Autodesk Inventor part; units mm, degrees
ref_plane "YZ Plane" through (0, 0, 0) normal (1, 0, 0) x (0, 1, 0)
ref_plane "XZ Plane" through (0, 0, 0) normal (0, 1, 0) x (-1, 0, 0)
ref_plane "XY Plane" through (0, 0, 0) normal (0, 0, 1) x (1, 0, 0)
sketch "Sketch1" plane through (0, 0, 0) normal (0, 0, 1) x (1, 0, 0)
  line L0 (-4.3614, 7.1036) -> (6.1386, 7.1036)
  line L1 (6.1386, 7.1036) -> (6.1386, -5.3964)
  line L2 (-4.3614, -5.3964) -> (-4.3614, 7.1036)
  line L3 (-4.3614, -5.3964) -> (-17.0614, -5.3964)
  line L4 (-4.3614, -5.3964) -> (8.3386, -5.3964) construction
  line L5 (-17.0614, -5.3964) -> (-17.0614, 12.1836)
  line L6 (-17.0614, 12.1836) -> (18.8386, 12.1836)
  line L7 (18.8386, 12.1836) -> (18.8386, -5.3964)
  line L8 (18.8386, -5.3964) -> (6.1386, -5.3964)
  point P0 (0, 0)
  dimension "d0" = 10.5
  dimension "d1" = 12.5
  dimension "d2" = 12.7
  dimension "d3" = 180
  dimension "d6" = 12.7
  dimension "d9" = 5.08
extrude "Extrusion1" add sketch "Sketch1" along normal blind 15
sketch "Sketch2" plane through (6.1386, -5.3964, 0) normal (0, -1, 0) x (1, 0, 0)
  circle A0 centre (6.35, 7.5) radius 3.175
  circle A1 centre (-16.85, 7.5) radius 3.175
  line L0 (0, 0) -> (12.7, 0)
  line L1 (-23.2, 0) -> (-23.2, 15)
  line L2 (-23.2, 15) -> (-10.5, 15)
  point P0 (-6.1386, 0)
  dimension "d12" = 6.35
  dimension "d13" = 6.35
  dimension "d14" = 7.5
  dimension "d15" = 6.35
  dimension "d16" = 6.35
  dimension "d17" = 7.5
extrude "Extrusion2" cut sketch "Sketch2" against normal blind 21.5125
properties part number "motor mount"
For this review, take the finished solid that the model builds, in its own axes (mm). A direction names the side the tool comes from. Round coordinates to 2 decimals unless told otherwise and drop trailing zeros. Write each loop counter-clockwise with the first axis right and the second up, starting at its lowest first coordinate (ties: lowest second). Pieces come first, ordered by that corner, then holes. Notation, with made-up numbers: (48, 29) - (52, 29) arc R9 ccw to (52, 41) - close; hole circle Ø6 at (10, 34). An arc over 180 degrees is marked (long way). Answer as a JSON object with one key per item and string values.
1. Draft analysis for pull direction Z (two halves, no side actions). For faces 3 (the face through (1, 12.184, 7)), 4 (the face through (0.6, 7.4, 15)), 5 (the face through (-7.78, 3.27, 6.28)), state which applies: +Z half, -Z half, draft (parallel to the pull), parting line (faces both ways), or undercut.
Response values:
{"face 3": "draft", "face 4": "+Z half", "face 5": "undercut"}
2. We need section A-A on y = 3.5. Give the boundary of the cut face in (x, z) (3 decimals), then the cut area to 3 significant figures.
Response values:
{"outline": "(-17.061, 0) - (-4.361, 0) - (-4.361, 15) - (-17.061, 15) - close; (6.139, 0) - (18.839, 0) - (18.839, 15) - (6.139, 15) - close; hole circle Ø6.35 at (-10.711, 7.5); hole circle Ø6.35 at (12.489, 7.5)", "area": "318 mm2"}
3. For pin 1 Ø5 at (x, z) = (12.49, 7.5) entering from +Y; pin 2 Ø8.5 at (x, z) = (1, 9.5) entering from -Y, all flat-tipped, find the tip position at first contact; note any pin that passes through.
Response values:
{"pin 1": "passes through", "pin 2": "stops at y = 7.1"}
4. We need section B-B on z = 7.5. Give the boundary of the cut face in (x, y).
Response values:
{"outline": "(-17.06, -5.4) - (-13.89, -5.4) - (-13.89, 12.18) - (-17.06, 12.18) - close; (-7.54, -5.4) - (-4.36, -5.4) - (-4.36, 7.1) - (6.14, 7.1) - (6.14, -5.4) - (9.31, -5.4) - (9.31, 12.18) - (-7.54, 12.18) - close; (15.66, -5.4) - (18.84, -5.4) - (18.84, 12.18) - (15.66, 12.18) - close"}
5. We need section D-D on z = 13.5. Give the boundary of the cut face in (x, y).
Response values:
{"outline": "(-17.06, -5.4) - (-4.36, -5.4) - (-4.36, 7.1) - (6.14, 7.1) - (6.14, -5.4) - (18.84, -5.4) - (18.84, 12.18) - (-17.06, 12.18) - close"}
6. To check wall thickness, follow line 1 along X through (y, z) = (4.25, 14); line 2 along X through (y, z) = (-0.25, 8); line 3 along X through (y, z) = (-2.5, 9). State the ranges of each line that lie inside material, in increasing order.
Response values:
{"line 1": "x = -17.06 to -4.36, 6.14 to 18.84", "line 2": "x = -17.06 to -13.85, -7.58 to -4.36, 6.14 to 9.35, 15.62 to 18.84", "line 3": "x = -17.06 to -13.51, -7.91 to -4.36, 6.14 to 9.69, 15.29 to 18.84"}
7. We need section C-C on x = 11. Give the boundary of the cut face in (y, z), then the cut area to 3 significant figures.
Response values:
{"outline": "(-5.4, 0) - (12.18, 0) - (12.18, 4.7) - (-5.4, 4.7) - close; (-5.4, 10.3) - (12.18, 10.3) - (12.18, 15) - (-5.4, 15) - close", "area": "165 mm2"}
8. Tool access review of faces 1 (the face through (0.6, 7.4, 0)), 2 (the face through (6.139, 1, 7)): name each direction out of +Z, -Z, +X, -X, +Y, -Y from which nothing blocks a thin tool from reaching the whole face with its end or side.
Response values:
{"face 1": "-Z, +X, -X, +Y, -Y", "face 2": "+Z, -Z, -Y"}
